Check sheet for the modelled part. Datum: model origin and axes. Units: mm. A direction names the side the tool comes from. Give positions to 0.01 mm unless a question says otherwise; leave off trailing zeros. Order: outer loops, then holes, each group sorted by start corner. A loop starts at its lowest first (then second) coordinate and runs counter-clockwise, first axis right, second up.
from build123d import *

# Parameters (mm, degrees)
BOSS_EXTRU_1_DEPTH                             = 4
BOSS_EXTRU_2_DEPTH                             = 8
ENL_V_START                                    = -2
ESQUISSE3_R                                    = 10.25
ENL_V_MAT_EXTRU_1_DEPTH                        = 2
ESQUISSE6_R                                    = 2
ENL_V_MAT_EXTRU_2_DEPTH                        = 40.462007045
ESQUISSE7_R                                    = 8
BOSS_EXTRU_5_DEPTH                             = 16
ENL_V_MAT_EXTRU_3_DEPTH                        = 51.786317055
ENL_V_MAT_EXTRU_3_DEPTH_BACK                   = 51.786317055
ESQUISSE9_W                                    = 0.5
ESQUISSE9_H                                    = 9.601810628
FRAISAGE_POUR_VIS_T_TE_FRAIS_E_M31_D           = 3.4
FRAISAGE_POUR_VIS_T_TE_FRAIS_E_M31_DEPTH       = 8
FRAISAGE_POUR_VIS_T_TE_FRAIS_E_M31_CSINK_D     = 6.3
FRAISAGE_POUR_VIS_T_TE_FRAIS_E_M31_CSINK_ANGLE = 90


with BuildPart() as part:
    # Esquisse1 → Boss.-Extru.1 (new body)
    with BuildSketch(Plane.XY):
        with BuildLine():
            Line((25, -10), (25, 10))
            Line((25, 10), (19.364230348, 10))
            ThreePointArc((19.364230348, 10), (18.046020427, 10.546020427), (17.5, 11.864230348))
            Line((17.5, 11.864230348), (17.5, 13))
            ThreePointArc((17.5, 13), (14, 16.5), (10.5, 13))
            Line((10.5, 13), (10.5, 11.864230348))
            ThreePointArc((10.5, 11.864230348), (9.953979573, 10.546020427), (8.635769652, 10))
            Line((8.635769652, 10), (-9.635769652, 10))
            ThreePointArc((-9.635769652, 10), (-10.953979573, 10.546020427), (-11.5, 11.864230348))
            Line((-11.5, 11.864230348), (-11.5, 13))
            ThreePointArc((-11.5, 13), (-15, 16.5), (-18.5, 13))
            Line((-18.5, 13), (-18.5, 11.864230348))
            ThreePointArc((-18.5, 11.864230348), (-19.046020427, 10.546020427), (-20.364230348, 10))
            Line((-20.364230348, 10), (-25, 10))
            Line((-25, 10), (-25, -10))
            Line((-25, -10), (-20.364230348, -10))
            ThreePointArc((-20.364230348, -10), (-19.046020427, -10.546020427), (-18.5, -11.864230348))
            Line((-18.5, -11.864230348), (-18.5, -13))
            ThreePointArc((-18.5, -13), (-15, -16.5), (-11.5, -13))
            Line((-11.5, -13), (-11.5, -11.864230348))
            ThreePointArc((-11.5, -11.864230348), (-10.953979573, -10.546020427), (-9.635769652, -10))
            Line((-9.635769652, -10), (8.635769652, -10))
            ThreePointArc((8.635769652, -10), (9.953979573, -10.546020427), (10.5, -11.864230348))
            Line((10.5, -11.864230348), (10.5, -13))
            ThreePointArc((10.5, -13), (14, -16.5), (17.5, -13))
            Line((17.5, -13), (17.5, -11.864230348))
            ThreePointArc((17.5, -11.864230348), (18.046020427, -10.546020427), (19.364230348, -10))
            Line((19.364230348, -10), (25, -10))
        make_face()
    extrude(amount=BOSS_EXTRU_1_DEPTH)

    # Esquisse2 → Boss.-Extru.2 (add)
    with BuildSketch(Plane.ZY.offset(25)):
        with BuildLine():
            Line((-3.638732785, 12.740569992), (5.045284633, 11.827842982))
            ThreePointArc((5.045284633, 11.827842982), (11.431448255, 8.573930092), (14, 1.882624029))
            Line((14, 1.882624029), (14, -1.882624029))
            ThreePointArc((14, -1.882624029), (11.431448255, -8.573930092), (5.045284633, -11.827842982))
            Line((5.045284633, -11.827842982), (-3.638732785, -12.740569992))
            ThreePointArc((-3.638732785, -12.740569992), (-13.25, 0), (-3.638732785, 12.740569992))
        make_face()
    extrude(amount=BOSS_EXTRU_2_DEPTH)

    # Esquisse3 → Enlèv. mat.-Extru.1 (cut)
    with BuildSketch(Plane.ZY.offset(33).offset(ENL_V_START)):
        Circle(ESQUISSE3_R)
    extrude(amount=ENL_V_MAT_EXTRU_1_DEPTH, mode=Mode.SUBTRACT)

    # Esquisse6 → Enlèv. mat.-Extru.2 (cut, through all)
    with BuildSketch(Plane(origin=(0, 0, 0), x_dir=(-1, 0, 0), z_dir=(0, 0, -1))):
        with Locations((15, -13)):
            Circle(ESQUISSE6_R)
        with Locations((-14, -13)):
            Circle(ESQUISSE6_R)
        with Locations((-14, 13)):
            Circle(ESQUISSE6_R)
        with Locations((15, 13)):
            Circle(ESQUISSE6_R)
    extrude(amount=-ENL_V_MAT_EXTRU_2_DEPTH, mode=Mode.SUBTRACT)

    # Esquisse7 → Boss.-Extru.5 (add)
    with BuildSketch(Plane(origin=(25, 0, 0), x_dir=(0, 0, -1), z_dir=(1, 0, 0))):
        with Locations(Location((0, 0, 0), (0, 0, 120))):
            Circle(ESQUISSE7_R)
    extrude(amount=BOSS_EXTRU_5_DEPTH)

    # Esquisse9 → Enlèv. mat.-Extru.3 (cut, two sides: drawn at the far end of the back side and taken through both)
    with BuildSketch(Plane(origin=(0, 10, 0), x_dir=(1, 0, 0), z_dir=(0, 1, 0)).offset(-ENL_V_MAT_EXTRU_3_DEPTH_BACK)):
        with Locations((25.25, 4.800905314)):
            Rectangle(ESQUISSE9_W, ESQUISSE9_H)
    extrude(amount=ENL_V_MAT_EXTRU_3_DEPTH + ENL_V_MAT_EXTRU_3_DEPTH_BACK, mode=Mode.SUBTRACT)

    # Fraisage pour vis à tête fraisée M31
    with Locations(Plane(origin=(-25, 0, 0), x_dir=(0, 0, -1), z_dir=(1, 0, 0))):
        with Locations((-7.5, 0), (7.5, 0)):
            CounterSinkHole(FRAISAGE_POUR_VIS_T_TE_FRAIS_E_M31_D / 2, FRAISAGE_POUR_VIS_T_TE_FRAIS_E_M31_CSINK_D / 2, depth=FRAISAGE_POUR_VIS_T_TE_FRAIS_E_M31_DEPTH, counter_sink_angle=FRAISAGE_POUR_VIS_T_TE_FRAIS_E_M31_CSINK_ANGLE)


solid = part.part
1) Draft check along X on faces 4 (the face through (-28.76, -1.03, 6.15)), 5 (the face through (25, -9, 2)), 6 (the face through (13.9, -16.5, 2)). Enter one of: +X half, -X half, draft (parallel to the pull), parting line (faces both ways), or undercut.
Recorded:
face 4: draft
face 5: +X half
face 6: undercut
2) Depth check by flat-ended pin: pin 1 Ø1 at (y, z) = (-8, -8) entering from +X; pin 2 Ø5 at (x, y) = (-23.5, 10.5) entering from -Z; pin 3 Ø1.5 at (x, y) = (-25.5, 7.5) entering from +Z. Enter the tip coordinate at first touch or a pass-through.
Recorded:
pin 1: stops at x = -25
pin 2: stops at z = -10.16
pin 3: stops at z = 12.74
3) Section check C-C, the plane z = 2. State how many separate pieces and enclosed holes the cut face has, then the cut area to 3 significant figures.
Recorded:
separate pieces: 1
enclosed holes: 4
area: 1,520 mm2
4) Section check B-B, the plane y = 14. Record the cut outline in (x, z).
Recorded:
outline: (-18.35, 0) - (-16.73, 0) - (-16.73, 4) - (-18.35, 4) - close; (-13.27, 0) - (-11.65, 0) - (-11.65, 4) - (-13.27, 4) - close; (10.65, 0) - (12.27, 0) - (12.27, 4) - (10.65, 4) - close; (15.73, 0) - (17.35, 0) - (17.35, 4) - (15.73, 4) - close
5) Section check D-D, the plane x = 1. Record the cut outline in (y, z), then the cut area to 3 significant figures.
Recorded:
outline: (-10, 0) - (10, 0) - (10, 4) - (-10, 4) - close
area: 80.0 mm2
6) Section check A-A, the plane x = 14. Record the cut outline in (y, z), then the cut area to 3 significant figures.
Recorded:
outline: (-16.5, 0) - (-15, 0) - (-15, 4) - (-16.5, 4) - close; (-11, 0) - (11, 0) - (11, 4) - (-11, 4) - close; (15, 0) - (16.5, 0) - (16.5, 4) - (15, 4) - close
area: 100 mm2
7) Material ranges on L1, parallel to Z at x = -27.4, y = 0; L2, parallel to Y at x = 14, z = 1; L3, parallel to X at y = 5, z = 9.25, recorded low to high.
Recorded:
L1: z = -13.25 to -9.2, -5.8 to 5.8, 9.2 to 14
L2: y = -16.5 to -15, -11 to 11, 15 to 16.5
L3: x = -33 to -25
8) Set-up check for faces 1 (the face through (9.94, -10.53, 1.97)), 2 (the face through (-31, 0, 0)), 3 (the face through (-28.94, -12.28, 0.76)): record each of +Z, -Z, +X, -X, +Y, -Y from which the full face is reachable in a straight line by a thin tool's end or side.
Recorded:
face 1: +Z, -Z, -Y
face 2: -X
face 3: +Z, -X, -Y
